Read the model definition and answer for the solid it produces. Units are mm, in the model's axes. A direction names the side the tool comes from. Coordinates: 2 decimals unless noted, no trailing zeros. Order: outer loops, then holes, each group sorted by start corner. A loop starts at its lowest first (then second) coordinate and runs counter-clockwise, first axis right, second up. Notation, with made-up numbers: (43, 84) -> (86, 84) arc R17 cw to (86, 108) -> close; hole circle Ø1 at (5, 45.25). An arc over 180 degrees is marked (long way). Use CSV: the item, a comma, the result in double quotes.
```python
from build123d import *

# Parameters (mm, degrees)
SKETCH_1_R          = 3
EXTRUDE_1_DEPTH     = 12
SKETCH_2_R          = 1.25
CUT_EXTRUDE_1_DEPTH = 6


with BuildPart() as part:
    # ｽｹｯﾁ1 → ﾎﾞｽ - 押し出し1 (new, symmetric)
    with BuildSketch(Plane.XY):
        Circle(SKETCH_1_R)
    extrude(amount=EXTRUDE_1_DEPTH, both=True)

    # ｽｹｯﾁ2 → ｶｯﾄ - 押し出し1 (cut)
    with BuildSketch(Plane.XY.offset(12)):
        Circle(SKETCH_2_R)
    cut_extrude_1 = extrude(amount=-CUT_EXTRUDE_1_DEPTH, mode=Mode.SUBTRACT)

    # ﾐﾗｰ1: ｶｯﾄ - 押し出し1 across plane
    add(cut_extrude_1.mirror(Plane.XY), mode=Mode.SUBTRACT)


solid = part.part
```
Item 1: Straight lines are drawn through the part: line 1 along Y through (x, z) = (0, -7.95); line 2 along Z through (x, y) = (-0.05, 0.8); line 3 along X through (y, z) = (-0.6, -7). For each, find the intervals that lie inside material, in ascending order.
Return value:
line 1,"y = -3 to -1.25, 1.25 to 3"
line 2,"z = -6 to 6"
line 3,"x = -2.94 to -1.1, 1.1 to 2.94"
Item 2: A tool of negligible diameter and unlimited length cuts with its end or side. For faces 5 (the flat face through (0, 0, -6)), 6 (the flat face through (1, -1, -12)), from which of +Z, -Z, +X, -X, +Y, -Y can it reach the whole face along a straight path? Write none if from no direction.
Return value:
face 5,"-Z"
face 6,"-Z, +X, -X, +Y, -Y"
Item 3: Each of these flat-tipped pins is pushed along its axis until it touches: P1, Ø1, axis at x = 1.5, z = -7, coming from the -Y side; P2, Ø2, axis at x = 0, y = 0, coming from the +Z side; P3, Ø2, axis at x = 0, y = 0, coming from the -Z side. Where does it stop, or does it pass through?
Return value:
P1,"stops at y = -2.83"
P2,"stops at z = 6"
P3,"stops at z = -6"
Item 4: Find section D-D, the plane z = -0.75. Give the vertices of the cut face in (x, y), then the cut area to 3 significant figures.
Return value:
outline,"circle Ø6 at (0, 0)"
area,"28.3 mm^2"
Item 5: The mould has two halves that part along X. Classify faces 1 (the cylindrical face through (-3, 0, 0)), 2 (the flat face through (1, -1, 12)), 3 (the cylindrical face through (-0.27, -1.22, 9.04)), 4 (the flat face through (0, 0, 6)): +X half, -X half, draft (parallel to the pull), parting line (faces both ways), or undercut.
Return value:
face 1,"parting line"
face 2,"draft"
face 3,"undercut"
face 4,"undercut"
Item 6: Find section C-C, the plane z = 6.25. Give the vertices of the cut face in (x, y).
Return value:
outline,"circle Ø6 at (0, 0); hole circle Ø2.5 at (0, 0)"
Item 7: Find section A-A, the plane x = 0. Give the vertices of the cut face in (y, z).
Return value:
outline,"(-3, -12) -> (-1.25, -12) -> (-1.25, -6) -> (1.25, -6) -> (1.25, -12) -> (3, -12) -> (3, 12) -> (1.25, 12) -> (1.25, 6) -> (-1.25, 6) -> (-1.25, 12) -> (-3, 12) -> close"
